The model under review builds one solid part; all positions refer to its coordinate system, in mm. A direction names the side the tool comes from. Coordinates: 2 decimals unless noted, no trailing zeros. Loops run counter-clockwise (first coordinate to the right, second up) from the corner with the lowest first, then second, coordinate; pieces in that order, holes last. Notation, with made-up numbers: M 26,-22.5 L 63,-22.5 A31 cw 63,14.5 Z; hole C 61,7.25 d4. An arc over 180 degrees is marked long. One line per item, written item: value.
Autodesk Inventor part; units mm, degrees
ref_plane "YZ Plane" through (0, 0, 0) normal (1, 0, 0) x (0, 1, 0)
ref_plane "XZ Plane" through (0, 0, 0) normal (0, 1, 0) x (-1, 0, 0)
ref_plane "XY Plane" through (0, 0, 0) normal (0, 0, 1) x (1, 0, 0)
sketch "Sketch1" plane through (0, 0, 0) normal (0, 0, 1) x (1, 0, 0)
  line L0 (0, 0) -> (50.8, 0)
  line L1 (50.8, 0) -> (50.8, 50.8)
  line L2 (50.8, 50.8) -> (0, 50.8)
  line L3 (0, 50.8) -> (0, 0)
  dimension "d0" = 50.8
  dimension "d1" = 50.8
extrude "Extrusion1" add sketch "Sketch1" along normal blind 50.8
sketch "Sketch2" plane through (0, 0, 50.8) normal (0, 0, 1) x (1, 0, 0)
  line L0 (0, 50.8) -> (44.45, 50.8)
  line L1 (44.45, 50.8) -> (44.45, 6.35)
  line L2 (44.45, 6.35) -> (0, 6.35)
  line L3 (0, 6.35) -> (0, 50.8)
  point P0 (0, 0)
  dimension "d4" = 44.45
  dimension "d5" = 44.45
extrude "Extrusion2" cut sketch "Sketch2" against normal blind 152.4
fillet "Fillet1" radius 3.175 1 edges at (44.45, 6.35, 25.4)
sketch "Sketch3" plane through (44.45, 50.8, 0) normal (-1, 0, 0) x (0, 0, 1)
  circle A0 centre (25.4, -20.6375) radius 4.7625
  line L0 (0, -41.275) -> (0, 0)
  line L1 (0, 0) -> (50.8, 0)
  point P0 (0, -50.8)
  dimension "d9" = 9.525
  dimension "d10" = 25.4
  dimension "d11" = 20.6375
extrude "Extrusion3" cut sketch "Sketch3" against normal blind 152.4
sketch "Sketch4" plane through (0, 6.35, 50.8) normal (0, 1, 0) x (1, 0, 0)
  line L0 (0, 50.8) -> (41.275, 50.8)
  line L1 (0, 0) -> (0, 50.8)
  point P0 (20.6375, 38.1)
  point P1 (20.6375, 12.7)
  dimension "d14" = 25.4
  dimension "d15" = 12.7
  dimension "d16" = 20.6375
  dimension "d17" = 20.6375
hole "Hole1" at (20.6375, 6.35, 12.7) at (20.6375, 6.35, 38.1) direction (0, -1, 0) diameter 6.35 end through all
properties part number "clevece plate"
(1) Add section A-A on z = 25.4. State the section outline as (x, y) points (3 decimals).
Checks:
outline: M 0,0 L 50.8,0 L 50.8,25.4 L 44.45,25.4 L 44.45,9.525 A3.175 cw 41.275,6.35 L 0,6.35 Z; M 44.45,34.925 L 50.8,34.925 L 50.8,50.8 L 44.45,50.8 Z
(2) Draft analysis for pull direction Y (two halves, no side actions). For faces 1 (the face through (50.8, 25, 25)), 2 (the face through (25, 0, 25)), 3 (the face through (47.581, 34.884, 24.78)), state which applies: pulls with the +Y half, pulls with the -Y half, needs draft (parallel to the pull), parting line crosses it, or undercut.
Checks:
face 1: needs draft
face 2: pulls with the -Y half
face 3: undercut
(3) Tool access review of faces 4 (the face through (21, 6.35, 26)), 5 (the face through (23.737, 3.131, 12.012)): name each direction out of +Z, -Z, +X, -X, +Y, -Y from which nothing blocks a thin tool from reaching the whole face with its end or side.
Checks:
face 4: +Z, -Z, -X, +Y
face 5: +Y, -Y
(4) To check wall thickness, follow L1, parallel to X at y = 1, z = 38; L2, parallel to Y at x = 49.5, z = 25.4 (3 decimals); L3, parallel to X at y = 20.5, z = 15.5. State the ranges of each line that lie inside material, in increasing order. Write a range as [from, to].
Checks:
L1: [0, 17.46], [23.81, 50.8]
L2: [0, 25.4], [34.925, 50.8]
L3: [44.45, 50.8]
(5) Add section B-B on x = 47.5. State the section outline as (y, z) points (1 decimal).
Checks:
outline: M 0,0 L 50.8,0 L 50.8,50.8 L 0,50.8 Z; hole C 30.2,25.4 d9.5
(6) Add section D-D on x = 21.5. State the section outline as (y, z) points.
Checks:
outline: M 0,0 L 6.35,0 L 6.35,9.64 L 0,9.64 Z; M 0,15.76 L 6.35,15.76 L 6.35,35.04 L 0,35.04 Z; M 0,41.16 L 6.35,41.16 L 6.35,50.8 L 0,50.8 Z
(7) Insertion check: pin 1 Ø1 at (x, z) = (7, 20) entering from +Y. The pin has a flat end and moves straight along its axis. Give the tip position at first contact, or say it passes through.
Checks:
pin 1: y = 6.35
